Could you check a few things on this drawing? It's one solid part, dimensions in mm from its lowest x, y, z. Round coordinates to 2 decimals unless told otherwise and drop trailing zeros. Write each loop counter-clockwise with the first axis right and the second up, starting at its lowest first coordinate (ties: lowest second). Pieces come first, ordered by that corner, then holes. Notation, with made-up numbers: (-9, -23) -> (18, -23) arc R14 cw to (18, -19) -> close; hole circle Ø4 at (-10, 22). An arc over 180 degrees is marked (long way). Answer in a Markdown table with one row per item.
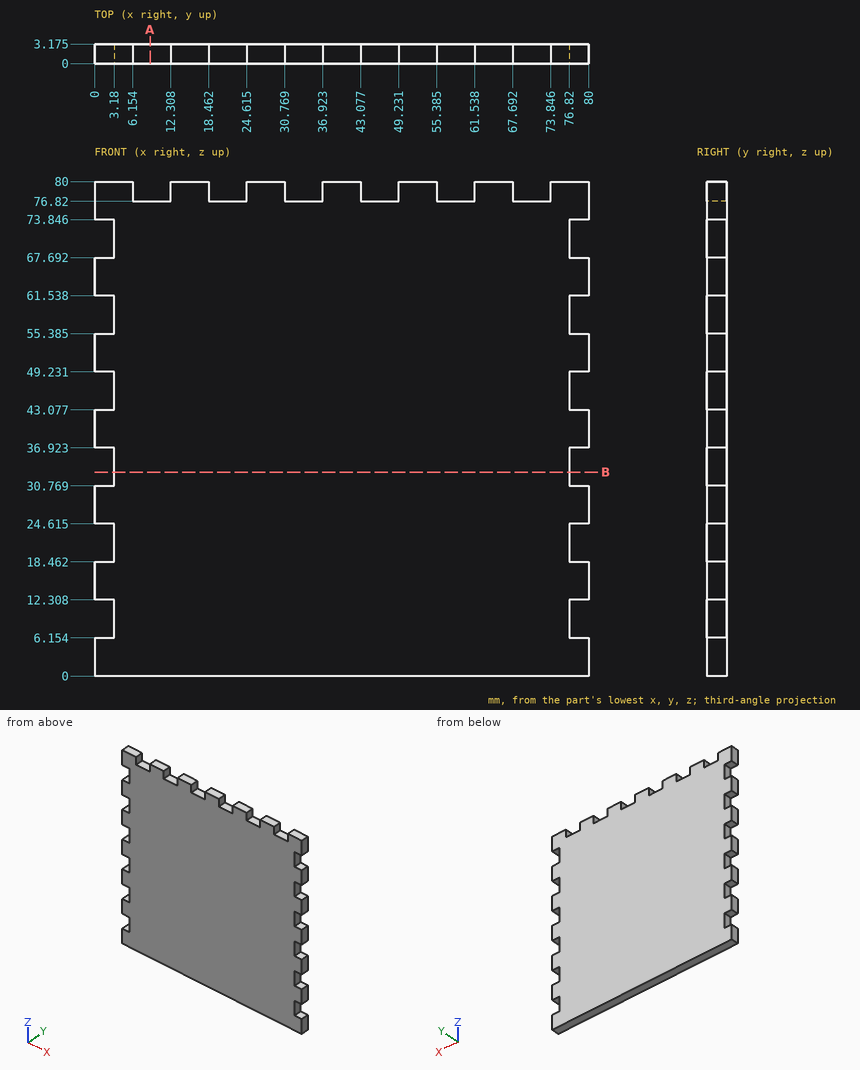
1) For pin 1 (1.6 mm diameter, centred on y = 1, z = 44.5, fed in from +X); pin 2 (1 mm diameter, centred on y = 2, z = 58.5, fed in from -X); pin 3 (1.5 mm diameter, centred on x = 34.5, y = 1.5, fed in from +Z), each with a flat end and sliding along its axis, tell me the tip position at first contact or that it passes through.
Response:
| item | result |
|---|---|
| pin 1 | stops at x = 76.82 |
| pin 2 | stops at x = 3.18 |
| pin 3 | stops at z = 76.82 |
2) I want a section at B-B, the plane z = 33. List the corners of the cut face in (x, y) for me (1 decimal).
Response:
| item | result |
|---|---|
| outline | (3.2, 0) -> (76.8, 0) -> (76.8, 3.2) -> (3.2, 3.2) -> close |
3) I want a section at A-A, the plane x = 9. List the corners of the cut face in (y, z) for me (1 decimal).
Response:
| item | result |
|---|---|
| outline | (0, 0) -> (3.2, 0) -> (3.2, 76.8) -> (0, 76.8) -> close |
4) I need wall thicknesses on line 1 (Z direction, x = 61.5, y = 0.35); line 2 (X direction, y = 1.05, z = 55.5). Which ranges of each line are inside material? Lowest first, please. Write a range as [from, to].
Response:
| item | result |
|---|---|
| line 1 | z = [0, 76.82] |
| line 2 | x = [3.18, 76.82] |
